from build123d import *

# Parameters (mm, degrees)
BOSS_EXTRUDE1_DEPTH = 50
SHELL2_T            = -2
CUT_EXTRUDE1_DEPTH  = 60


with BuildPart() as part:
    # Sketch1 → Boss-Extrude1 (new body)
    with BuildSketch(Plane.XY):
        Polygon((-100, 25), (-75, 0), (0, 0), (0, 50), (-100, 50), align=None)
        with BuildLine():
            ThreePointArc((-75, 21.327014218), (-78.672985782, 25), (-75, 28.672985782))
            Line((-75, 28.672985782), (-20.142180095, 28.672985782))
            ThreePointArc((-20.142180095, 28.672985782), (-16.469194313, 25), (-20.142180095, 21.327014218))
            Line((-20.142180095, 21.327014218), (-75, 21.327014218))
        make_face(mode=Mode.SUBTRACT)
    extrude(amount=BOSS_EXTRUDE1_DEPTH)

    # Shell2
    shell2_openings = [part.faces().sort_by_distance(p)[0] for p in [
        (-87.5, 12.5, 25),
        (-37.5, 0, 25),
        (-50, 50, 25),
        (-100, 37.5, 25),
        (-78.672985782, 25, 25),
        (-47.571090047, 28.672985782, 25),
        (-16.469194313, 25, 25),
        (-47.571090047, 21.327014218, 25),
        (-86.709430585, 13.290569415, 0),
    ]]
    offset(amount=SHELL2_T, openings=shell2_openings, kind=Kind.INTERSECTION)

    # Sketch2 → Cut-Extrude1 (cut)
    with BuildSketch(Plane(origin=(0, 0, 0), x_dir=(0, 0, -1), z_dir=(1, 0, 0))):
        with BuildLine():
            Line((-40, 27.5), (-10, 27.5))
            ThreePointArc((-10, 27.5), (-7.5, 25), (-10, 22.5))
            Line((-10, 22.5), (-40, 22.5))
            ThreePointArc((-40, 22.5), (-42.5, 25), (-40, 27.5))
        make_face()
    extrude(amount=-CUT_EXTRUDE1_DEPTH, mode=Mode.SUBTRACT)


solid = part.part
Verification items for the finished model (mm, model axes). A direction names the side the tool comes from. Coordinates: 2 decimals unless noted, no trailing zeros. Order: outer loops, then holes, each group sorted by start corner. A loop starts at its lowest first (then second) coordinate and runs counter-clockwise, first axis right, second up. Notation, with made-up numbers: M 33,72.25 L 37,72.25 A25 ccw 37,84.25 Z; hole C 21,-3.75 d3. An arc over 180 degrees is marked long. One line per item, written item: value. Start each with the question number.
Item 1: Sectioned sample at B-B (x = -28). Enter the section's corners in (y, z), then the cut area to 3 significant figures.
Item 2: Access from +Z, -Z, +X, -X, +Y, -Y to the whole of each face (thin tool, end or side, straight path). Record for faces 1 (the flat face through (-48, 28.673, 49)), 2 (the flat face through (-1, 22.5, 25)), 3 (the flat face through (-2, 19, 24)).
Item 3: Sectioned sample at D-D (z = 3). Enter the section's corners in (x, y).
Item 4: Sectioned sample at A-A (z = 23). Enter the section's corners in (x, y), then the cut area to 3 significant figures.
Item 5: Mould release check, pull along X, two halves, no side actions. Record for faces 4 (the flat face through (-88, 13, 49)), 5 (the cylindrical face through (-78.672, 24.919, 48.986)), 6 (the cylindrical face through (-1, 24.9, 42.5)): released by +X, released by -X, zero draft, split by the parting line, or undercut.
Item 6: Scan lines: probe 1 along X at (y, z) = (31, 2); probe 2 along Z at (x, y) = (-34, 21). Record each from-to range of solid material in increasing order.
Item 7: Gauge pin test, flat ends, axial feed: pin 1 (8 mm diameter, centred on y = 24, z = 42.5, fed in from -X); pin 2 (1 mm diameter, centred on x = -63, y = 38, fed in from -Z); pin 3 (2 mm diameter, centred on y = 25, z = 14.5, fed in from -X). Record the tip position at first contact, or that the pin passes through.
Item 8: Sectioned sample at C-C (y = 15). Enter the section's corners in (x, z), then the cut area to 3 significant figures.
Conclusion:
1. outline: M 0,48 L 21.33,48 L 21.33,50 L 0,50 Z; M 28.67,48 L 50,48 L 50,50 L 28.67,50 Z
1. area: 85.3 mm^2
2. face 1: +Z, -Z
2. face 2: +X, -X
2. face 3: -Z, -X, +Y, -Y
3. outline: M -2,0 L 0,0 L 0,50 L -2,50 Z
4. outline: M -2,0 L 0,0 L 0,22.5 L -2,22.5 Z; M -2,27.5 L 0,27.5 L 0,50 L -2,50 Z
4. area: 90.0 mm^2
5. face 4: released by -X
5. face 5: undercut
5. face 6: zero draft
6. probe 1: x = -2 to 0
6. probe 2: z = 48 to 50
7. pin 1: stops at x = -2
7. pin 2: stops at z = 48
7. pin 3: passes through
8. outline: M -90,48 L -2,48 L -2,0 L 0,0 L 0,50 L -90,50 Z
8. area: 276 mm^2
